```python
from build123d import *

# Parameters (mm, degrees)
F0_R     = 16.891
F0_R_2   = 1.905
F1_DEPTH = 2.032
F2_R     = 0.635
F0_R_3   = 19.05
F3_DEPTH = 2.54
F4_R     = 1.27


with BuildPart() as f1:
    # F0 (on Front) → F1 (new body)
    with BuildSketch(Plane.XZ):
        Circle(F0_R)
        with Locations((-6.35, -6.35)):
            Circle(F0_R_2, mode=Mode.SUBTRACT)
        with Locations((6.35, -6.35)):
            Circle(F0_R_2, mode=Mode.SUBTRACT)
        with Locations((-6.35, 6.35)):
            Circle(F0_R_2, mode=Mode.SUBTRACT)
        with Locations((6.35, 6.35)):
            Circle(F0_R_2, mode=Mode.SUBTRACT)
    extrude(amount=F1_DEPTH)

    # F2
    f2_edges = [f1.edges().sort_by_distance(p)[0] for p in [
        (-16.891, -2.032, 0),
        (-16.891, 0, 0),
    ]]
    fillet(f2_edges, radius=F2_R)

    # F0 (on Front) → F3 (join)
    with BuildSketch(Plane.XZ):
        Circle(F0_R_3)
        Circle(F0_R, mode=Mode.SUBTRACT)
    extrude(amount=F3_DEPTH)

    # F4
    f4_edges = [f1.edges().sort_by_distance(p)[0] for p in [
        (-19.05, -2.54, 0),
    ]]
    fillet(f4_edges, radius=F4_R)


solid = f1.part
```
Part model, mm, in its own coordinate system. A direction names the side the tool comes from. Give positions to 0.01 mm unless a question says otherwise; leave off trailing zeros. Write each loop counter-clockwise with the first axis right and the second up, starting at its lowest first coordinate (ties: lowest second). Pieces come first, ordered by that corner, then holes. Notation, with made-up numbers: (75, 82) -> (120, 82) arc R25 ccw to (120, 111) -> close; hole circle Ø6 at (63.25, 86.25). An arc over 180 degrees is marked (long way). Put each result on its own line as item: value. Start each with the question number.
Item 1: Which spindle directions (+Z, -Z, +X, -X, +Y, -Y) get a long thin tool onto all of the face, cutting with end or side? Do faces 5 (the face through (4.84, -1, 5.19)), 6 (the face through (0, -2.032, 0)). Say none if no direction does.
Item 2: Cut at A-A (z = 0). List the corners of the cut face in (x, y) (3 decimals), then the cut area to 3 significant figures.
Item 3: Wall check: L1, parallel to Z at x = -9, y = -0.2; L2, parallel to X at y = -0.75, z = -7.5; L3, parallel to Y at x = 10, z = -4.5. Give the ranges that are in metal, low to high. Write a range as [from, to].
Item 4: Pull direction X, two halves, no side cores. Call faces 1 (the face through (-15.12, -0.63, -11.59)), 2 (the face through (0, 0, 0)), 3 (the face through (-8.253, -1.002, 6.434)), 4 (the face through (-6.8, -1, -8.2)): pulls with the +X half, pulls with the -X half, needs draft (parallel to the pull), parting line crosses it, or undercut.
Item 5: Pin check, flat tips, straight feed: pin 1 Ø10 at (x, z) = (-2.5, 8.5) entering from -Y; pin 2 Ø12 at (x, z) = (-6, -11.5) entering from -Y; pin 3 Ø3 at (x, z) = (6.35, 6.35) entering from -Y; pin 4 Ø1 at (y, z) = (-0.5, 12.5) entering from +X. Stop position of each tip, or through.
Item 6: Cut at B-B (x = 5). State how many separate pieces and enclosed holes the cut face has, then the cut area to 3 significant figures.
Answer list:
1. face 5: +Y, -Y
1. face 6: -Y
2. outline: (-19.05, -1.27) arc R1.27 ccw to (-17.78, -2.54) -> (-16.891, -2.54) -> (-16.891, -1.397) arc R0.635 ccw to (-16.256, -2.032) -> (16.256, -2.032) arc R0.635 ccw to (16.891, -1.397) -> (16.891, -2.54) -> (17.78, -2.54) arc R1.27 ccw to (19.05, -1.27) -> (19.05, 0) -> (16.891, 0) -> (16.891, -0.635) arc R0.635 ccw to (16.256, 0) -> (-16.256, 0) arc R0.635 ccw to (-16.891, -0.635) -> (-16.891, 0) -> (-19.05, 0) -> close
2. area: 78.6 mm2
3. L1: z = [-16.79, -14.29], [-14.09, 14.09], [14.29, 16.79]
3. L2: x = [-17.51, -7.87], [-4.83, 4.83], [7.87, 17.51]
3. L3: y = [-2.03, 0]
4. face 1: parting line crosses it
4. face 2: needs draft
4. face 3: undercut
4. face 4: undercut
5. pin 1: stops at y = -2.03
5. pin 2: stops at y = -2.54
5. pin 3: passes through
5. pin 4: stops at x = 14.8
6. separate pieces: 3
6. enclosed holes: 0
6. area: 65.0 mm2
